Model file for the job. Use its own axes, mm. A direction names the side the tool comes from. Round coordinates to 2 decimals unless told otherwise and drop trailing zeros. Answer as CSV lines item,"result".
```python
from build123d import *

# Parameters (mm, degrees)
F1_DEPTH = 25.4


with BuildPart() as f1:
    # F0 (on Front) → F1 (new body, symmetric)
    with BuildSketch(Plane.XZ):
        with BuildLine():
            Line((-41.275, 9.525), (18.9229995012, 9.525))
            Line((18.9229995012, 9.525), (18.9229995012, 48.0189798517))
            ThreePointArc((18.9229995012, 48.0189798517), (27.5958880394, 69.7458014014), (48.8464394104, 79.5278173835))
            add(Edge.make_bspline(
                [(-41.275, 9.525), (-37.3546025083, 80.3186400557), (32.5938258146, 79.2506709796), (48.8464394104, 79.5278173835)],
                knots=[0, 0, 0, 0, 0.8264340186, 0.8264340186, 0.8264340186, 0.8264340186], degree=3))
        make_face()
        with BuildLine():
            Line((18.9229995012, 9.525), (41.275, 9.525))
            Line((41.275, 9.525), (41.275, 48.0189798517))
            ThreePointArc((41.275, 48.0189798517), (43.9692765801, 54.5235389122), (50.4738356406, 57.2178154923))
            Line((50.4738356406, 57.2178154923), (53.6273793955, 57.2178154923))
            Line((53.6273793955, 57.2178154923), (53.6273793955, 79.5951649401))
            add(Edge.make_bspline(
                [(50.4738356406, 79.5698159911), (52.5255819675, 79.6536185215), (52.860162183, 79.8598219744), (53.6273793955, 79.5951649401)],
                knots=[0.8581554272, 0.8581554272, 0.8581554272, 0.8581554272, 1, 1, 1, 1], degree=3))
            add(Edge.make_bspline(
                [(48.8464394104, 79.5278173835), (49.4702711805, 79.5384552253), (50.0149933862, 79.5510748137), (50.4738356406, 79.5698159911)],
                knots=[0.8264340186, 0.8264340186, 0.8264340186, 0.8264340186, 0.8581554272, 0.8581554272, 0.8581554272, 0.8581554272], degree=3))
            ThreePointArc((48.8464394104, 79.5278173835), (27.5958880394, 69.7458014014), (18.9229995012, 48.0189798517))
            Line((18.9229995012, 48.0189798517), (18.9229995012, 9.525))
        make_face()
    extrude(amount=F1_DEPTH, both=True)


solid = f1.part
```
Q1. Tool access for faces 1 (the flat face through (6, -25.4, 45)), 2 (the flat face through (52, 0, 57.218)): list every direction of +Z, -Z, +X, -X, +Y, -Y with a clear straight run to the whole face (end or side of a thin tool).
Checks:
face 1,"+Z, -Z, +X, -X, -Y"
face 2,"-Z, +X, +Y, -Y"
Q2. Wall check: L1, parallel to X at y = -18.5, z = 47 (1 decimal); L2, parallel to Z at x = 24, y = 15 (3 decimals); L3, parallel to Z at x = -21, y = -6.5 (3 decimals). Give the ranges that are in metal, low to high. Write a range as [from, to].
Checks:
L1,"[-30.1, 41.3]"
L2,"[9.525, 77.829]"
L3,"[9.525, 57.953]"
Q3. Flat gauge pins, fed straight in: pin 1 (0.9 mm diameter, centred on x = 52.5, y = 3.5, fed in from -Z); pin 2 (4 mm diameter, centred on y = -8, z = 29, fed in from -X); pin 3 (19 mm diameter, centred on y = 8.5, z = 38, fed in from +X) (3 decimals). Where does each tip first touch, or does it go through?
Checks:
pin 1,"z = 57.22"
pin 2,"x = -38.69"
pin 3,"x = 41.275"
